Geometry: see drawing. Coordinates: mm, zero at the bounding-box minimum. Round coordinates to 2 decimals unless told otherwise and drop trailing zeros. Write each loop counter-clockwise with the first axis right and the second up, starting at its lowest first coordinate (ties: lowest second). Pieces come first, ordered by that corner, then holes. Notation, with made-up numbers: (24, 40.5) -> (46, 40.5) arc R10 cw to (46, 56.5) -> close; hole circle Ø11 at (69.5, -37.5). An arc over 180 degrees is marked (long way). Use CSV: the item, a comma, the result in double quotes.
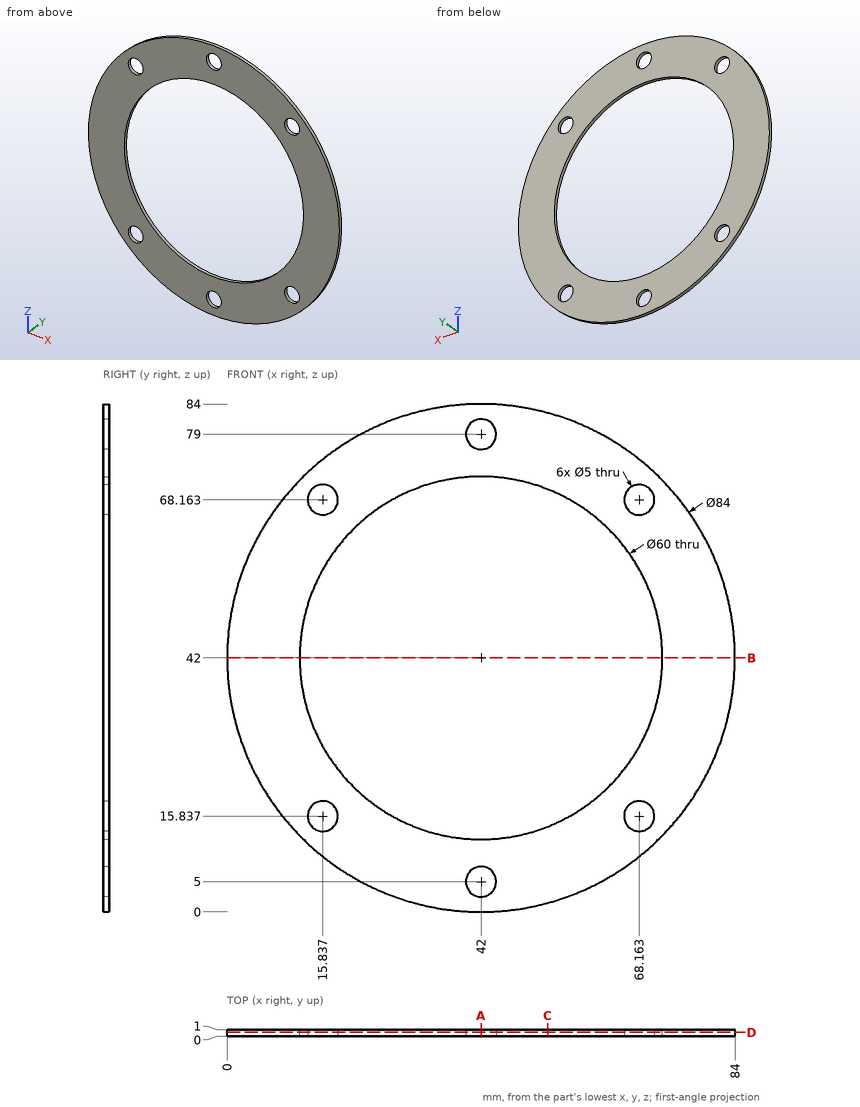
Item 1: Section query D-D on y = 0.6. Return the cut outline in (x, z), plus the area to 3 significant figures.
Worked answers:
outline,"circle Ø84 at (42, 42); hole circle Ø60 at (42, 42); hole circle Ø5 at (15.84, 15.84); hole circle Ø5 at (15.84, 68.16); hole circle Ø5 at (42, 5); hole circle Ø5 at (42, 79); hole circle Ø5 at (68.16, 15.84); hole circle Ø5 at (68.16, 68.16)"
area,"2,600 mm²"
Item 2: Line query: line 1 (Z direction, x = 42, y = 0.85); line 2 (X direction, y = 0.3, z = 42); line 3 (Z direction, x = 26, y = 0.7). Output: solid intervals per line, ascending.
Worked answers:
line 1,"z = 0 to 2.5, 7.5 to 12, 72 to 76.5, 81.5 to 84"
line 2,"x = 0 to 12, 72 to 84"
line 3,"z = 3.17 to 16.62, 67.38 to 80.83"
Item 3: Section query A-A on x = 42. Return the cut outline in (y, z).
Worked answers:
outline,"(0, 0) -> (1, 0) -> (1, 2.5) -> (0, 2.5) -> close; (0, 7.5) -> (1, 7.5) -> (1, 12) -> (0, 12) -> close; (0, 72) -> (1, 72) -> (1, 76.5) -> (0, 76.5) -> close; (0, 81.5) -> (1, 81.5) -> (1, 84) -> (0, 84) -> close"
Item 4: Section query C-C on x = 53. Return the cut outline in (y, z).
Worked answers:
outline,"(0, 1.47) -> (1, 1.47) -> (1, 14.09) -> (0, 14.09) -> close; (0, 69.91) -> (1, 69.91) -> (1, 82.53) -> (0, 82.53) -> close"
Item 5: First-contact query: pin 1 Ø1 at (x, z) = (62, 18) entering from -Y. Flat tip, straight axial feed; report the tip coordinate or a pass-through.
Worked answers:
pin 1,"stops at y = 0"
Item 6: Section query B-B on z = 42. Return the cut outline in (x, y).
Worked answers:
outline,"(0, 0) -> (12, 0) -> (12, 1) -> (0, 1) -> close; (72, 0) -> (84, 0) -> (84, 1) -> (72, 1) -> close"
